from build123d import *

# Parameters (mm, degrees)
BOSS_EXTRUDE1_DEPTH         = 2.54
F_11_0_191_DIAMETER_HOLE2_D = 4.8514
F_11_0_191_DIAMETER_HOLE3_D = 4.8514
SKETCH17_W                  = 6.35
SKETCH17_H                  = 50.8
SKETCH17_W_2                = 50.8
SKETCH17_H_2                = 6.35
SKETCH17_H_3                = 25.4
CUT_EXTRUDE12_DEPTH         = 304.883162745
MIRROR1_OUTLINE_W           = 6.35
MIRROR1_OUTLINE_H           = 50.8
MIRROR1_OUTLINE_R           = 2.4257
MIRROR1_OUTLINE_W_2         = 50.8
MIRROR1_OUTLINE_H_2         = 6.35
MIRROR1_DEPTH               = 2.54
SHELL1_START                = 0.1016
SHELL1_OUTLINE_W            = 545.8968
SHELL1_OUTLINE_H            = 393.4968
SHELL1_OUTLINE_W_2          = 51.0032
SHELL1_OUTLINE_H_2          = 6.5532
SHELL1_OUTLINE_W_3          = 6.5532
SHELL1_OUTLINE_H_3          = 51.0032
SHELL1_OUTLINE_R            = 2.5273
SHELL1_DEPTH                = 2.3368


# Read off the part's stored shape, not the designer's step: Mirror1, Shell1
with BuildPart() as part:
    # Sketch1 → Boss-Extrude1 (new body)
    with BuildSketch(Plane(origin=(0, 0, 0), x_dir=(1, 0, 0), z_dir=(0, 1, 0))):
        Polygon((0, 63.5), (-273.05, 63.5), (-273.05, -63.5), (-273.05, -133.35), (273.05, -133.35), (273.05, -63.5), (273.05, 63.5), align=None)
    extrude(amount=BOSS_EXTRUDE1_DEPTH)

    # #11 (0.191) Diameter Hole2 (through all)
    with Locations(Plane(origin=(0, 2.54, 0), x_dir=(1, 0, 0), z_dir=(0, 1, 0))):
        with Locations((-119.126, -56.127777467), (-38.862, -56.127777467), (38.862, -56.127777467), (119.126, -56.127777467)):
            Hole(F_11_0_191_DIAMETER_HOLE2_D / 2)

    # #11 (0.191) Diameter Hole3 (through all)
    with Locations(Plane(origin=(0, 2.54, 0), x_dir=(1, 0, 0), z_dir=(0, 1, 0))):
        with Locations((119.126, 63.5), (38.862, 63.5)):
            Hole(F_11_0_191_DIAMETER_HOLE3_D / 2)

    # Sketch17 → Cut-Extrude12 (cut, through all)
    with BuildSketch(Plane(origin=(0, 2.54, 0), x_dir=(1, 0, 0), z_dir=(0, 1, 0))):
        with Locations((-263.525, -57.15)):
            Rectangle(SKETCH17_W, SKETCH17_H)
        with Locations((-190.5, -123.825)):
            Rectangle(SKETCH17_W_2, SKETCH17_H_2)
        with Locations((190.5, -123.825)):
            Rectangle(SKETCH17_W_2, SKETCH17_H_2)
        with Locations((263.525, -57.15)):
            Rectangle(SKETCH17_W, SKETCH17_H)
        with Locations((0, -123.825)):
            Rectangle(SKETCH17_W_2, SKETCH17_H_2)
        with Locations((-263.525, 50.8)):
            Rectangle(SKETCH17_W, SKETCH17_H_3)
        with Locations((263.525, 50.8)):
            Rectangle(SKETCH17_W, SKETCH17_H_3)
    extrude(amount=-CUT_EXTRUDE12_DEPTH, mode=Mode.SUBTRACT)

    # Mirror1 outline → Mirror1 (add)
    with BuildSketch(Plane(origin=(0, 0, 0), x_dir=(1, 0, 0), z_dir=(0, 1, 0))):
        with BuildLine():
            Line((273.05, 63.5), (273.05, 260.35))
            Line((273.05, 260.35), (-273.05, 260.35))
            Line((-273.05, 260.35), (-273.05, 63.5))
            Line((-273.05, 63.5), (-266.7, 63.5))
            Line((-266.7, 63.5), (-266.7, 88.9))
            Line((-266.7, 88.9), (-260.35, 88.9))
            Line((-260.35, 88.9), (-260.35, 63.5))
            Line((-260.35, 63.5), (36.4363, 63.5))
            ThreePointArc((36.4363, 63.5), (38.862, 65.9257), (41.2877, 63.5))
            Line((41.2877, 63.5), (116.7003, 63.5))
            ThreePointArc((116.7003, 63.5), (119.126, 65.9257), (121.5517, 63.5))
            Line((121.5517, 63.5), (260.35, 63.5))
            Line((260.35, 63.5), (260.35, 88.9))
            Line((260.35, 88.9), (266.7, 88.9))
            Line((266.7, 88.9), (266.7, 63.5))
            Line((266.7, 63.5), (273.05, 63.5))
        make_face()
        with Locations((-263.525, 184.15)):
            Rectangle(MIRROR1_OUTLINE_W, MIRROR1_OUTLINE_H, mode=Mode.SUBTRACT)
        with Locations((-119.126, 183.127777467)):
            Circle(MIRROR1_OUTLINE_R, mode=Mode.SUBTRACT)
        with Locations((-38.862, 183.127777467)):
            Circle(MIRROR1_OUTLINE_R, mode=Mode.SUBTRACT)
        with Locations((-190.5, 250.825)):
            Rectangle(MIRROR1_OUTLINE_W_2, MIRROR1_OUTLINE_H_2, mode=Mode.SUBTRACT)
        with Locations((38.862, 183.127777467)):
            Circle(MIRROR1_OUTLINE_R, mode=Mode.SUBTRACT)
        with Locations((119.126, 183.127777467)):
            Circle(MIRROR1_OUTLINE_R, mode=Mode.SUBTRACT)
        with Locations((263.525, 184.15)):
            Rectangle(MIRROR1_OUTLINE_W, MIRROR1_OUTLINE_H, mode=Mode.SUBTRACT)
        with Locations((0, 250.825)):
            Rectangle(MIRROR1_OUTLINE_W_2, MIRROR1_OUTLINE_H_2, mode=Mode.SUBTRACT)
        with Locations((190.5, 250.825)):
            Rectangle(MIRROR1_OUTLINE_W_2, MIRROR1_OUTLINE_H_2, mode=Mode.SUBTRACT)
    extrude(amount=MIRROR1_DEPTH)

    # Shell1 outline → Shell1 (cut)
    with BuildSketch(Plane(origin=(0, 0, 0), x_dir=(1, 0, 0), z_dir=(0, 1, 0)).offset(SHELL1_START)):
        with Locations((0, 63.5)):
            Rectangle(SHELL1_OUTLINE_W, SHELL1_OUTLINE_H)
        with Locations((-190.5, -123.825)):
            Rectangle(SHELL1_OUTLINE_W_2, SHELL1_OUTLINE_H_2, mode=Mode.SUBTRACT)
        with Locations((-263.525, -57.15)):
            Rectangle(SHELL1_OUTLINE_W_3, SHELL1_OUTLINE_H_3, mode=Mode.SUBTRACT)
        with Locations((-119.126, -56.127777467)):
            Circle(SHELL1_OUTLINE_R, mode=Mode.SUBTRACT)
        with Locations((-38.862, -56.127777467)):
            Circle(SHELL1_OUTLINE_R, mode=Mode.SUBTRACT)
        with Locations((0, -123.825)):
            Rectangle(SHELL1_OUTLINE_W_2, SHELL1_OUTLINE_H_2, mode=Mode.SUBTRACT)
        with Locations((38.862, -56.127777467)):
            Circle(SHELL1_OUTLINE_R, mode=Mode.SUBTRACT)
        with Locations((119.126, -56.127777467)):
            Circle(SHELL1_OUTLINE_R, mode=Mode.SUBTRACT)
        with Locations((190.5, -123.825)):
            Rectangle(SHELL1_OUTLINE_W_2, SHELL1_OUTLINE_H_2, mode=Mode.SUBTRACT)
        with Locations((263.525, -57.15)):
            Rectangle(SHELL1_OUTLINE_W_3, SHELL1_OUTLINE_H_3, mode=Mode.SUBTRACT)
        with Locations((-263.525, 63.5)):
            Rectangle(SHELL1_OUTLINE_W_3, SHELL1_OUTLINE_H_3, mode=Mode.SUBTRACT)
        with Locations((-263.525, 184.15)):
            Rectangle(SHELL1_OUTLINE_W_3, SHELL1_OUTLINE_H_3, mode=Mode.SUBTRACT)
        with Locations((-190.5, 250.825)):
            Rectangle(SHELL1_OUTLINE_W_2, SHELL1_OUTLINE_H_2, mode=Mode.SUBTRACT)
        with Locations((-119.126, 183.127777467)):
            Circle(SHELL1_OUTLINE_R, mode=Mode.SUBTRACT)
        with Locations((-38.862, 183.127777467)):
            Circle(SHELL1_OUTLINE_R, mode=Mode.SUBTRACT)
        with Locations((38.862, 63.5)):
            Circle(SHELL1_OUTLINE_R, mode=Mode.SUBTRACT)
        with Locations((119.126, 63.5)):
            Circle(SHELL1_OUTLINE_R, mode=Mode.SUBTRACT)
        with Locations((263.525, 63.5)):
            Rectangle(SHELL1_OUTLINE_W_3, SHELL1_OUTLINE_H_3, mode=Mode.SUBTRACT)
        with Locations((38.862, 183.127777467)):
            Circle(SHELL1_OUTLINE_R, mode=Mode.SUBTRACT)
        with Locations((119.126, 183.127777467)):
            Circle(SHELL1_OUTLINE_R, mode=Mode.SUBTRACT)
        with Locations((0, 250.825)):
            Rectangle(SHELL1_OUTLINE_W_2, SHELL1_OUTLINE_H_2, mode=Mode.SUBTRACT)
        with Locations((263.525, 184.15)):
            Rectangle(SHELL1_OUTLINE_W_3, SHELL1_OUTLINE_H_3, mode=Mode.SUBTRACT)
        with Locations((190.5, 250.825)):
            Rectangle(SHELL1_OUTLINE_W_2, SHELL1_OUTLINE_H_2, mode=Mode.SUBTRACT)
    extrude(amount=SHELL1_DEPTH, mode=Mode.SUBTRACT)


solid = part.part
Verification items for the finished model (mm, model axes). Give positions to 0.01 mm unless a question says otherwise; leave off trailing zeros. Write each loop counter-clockwise with the first axis right and the second up, starting at its lowest first coordinate (ties: lowest second). Pieces come first, ordered by that corner, then holes. Notation, with made-up numbers: M 7.25,49 L 47.25,49 A19 cw 47.25,84 Z; hole C 30,22 d5. An arc over 180 degrees is marked long. Use CSV: the item, a comma, the result in double quotes.
1) Cross-section at D-D (x = 93.5). Enter the section's corners in (y, z), plus the area to 3 significant figures.
Final values:
outline,"M 0,-260.35 L 2.54,-260.35 L 2.54,133.35 L 0,133.35 Z; hole M 0.1,-260.25 L 2.44,-260.25 L 2.44,133.25 L 0.1,133.25 Z"
area,"80.5 mm²"
2) Cross-section at B-B (x = -173.5). Enter the section's corners in (y, z), plus the area to 3 significant figures.
Final values:
outline,"M 0,-260.35 L 2.54,-260.35 L 2.54,-254 L 0,-254 Z; M 0,-247.65 L 2.54,-247.65 L 2.54,120.65 L 0,120.65 Z; M 0,127 L 2.54,127 L 2.54,133.35 L 0,133.35 Z; hole M 0.1,-260.25 L 2.44,-260.25 L 2.44,-254.1 L 0.1,-254.1 Z; hole M 0.1,-247.55 L 2.44,-247.55 L 2.44,120.55 L 0.1,120.55 Z; hole M 0.1,127.1 L 2.44,127.1 L 2.44,133.25 L 0.1,133.25 Z"
area,"78.8 mm²"
3) Cross-section at C-C (z = 24). Enter the section's corners in (x, y), plus the area to 3 significant figures.
Final values:
outline,"M -273.05,0 L 273.05,0 L 273.05,2.54 L -273.05,2.54 Z; hole M -272.95,0.1 L 272.95,0.1 L 272.95,2.44 L -272.95,2.44 Z"
area,"111 mm²"
4) Go/stop test with a flat-tipped pin: pin 1 Ø1.5 at (x, z) = (-76.5, -163) entering from -Y. Record where the tip stops, or that it passes through.
Final values:
pin 1,"y = 0"
5) Cross-section at A-A (z = -74). Enter the section's corners in (x, y).
Final values:
outline,"M -273.05,0 L -266.7,0 L -266.7,2.54 L -273.05,2.54 Z; M -260.35,0 L 260.35,0 L 260.35,2.54 L -260.35,2.54 Z; M 266.7,0 L 273.05,0 L 273.05,2.54 L 266.7,2.54 Z; hole M -272.95,0.1 L -266.8,0.1 L -266.8,2.44 L -272.95,2.44 Z; hole M -260.25,0.1 L 260.25,0.1 L 260.25,2.44 L -260.25,2.44 Z; hole M 266.8,0.1 L 272.95,0.1 L 272.95,2.44 L 266.8,2.44 Z"
